Input: part model. Units: mm. Frame: model coordinates. A direction names the side the tool comes from. Coordinates: 2 decimals unless noted, no trailing zeros. Order: outer loops, then holes, each group sorted by start corner. A loop starts at its lowest first (then second) coordinate and runs counter-clockwise, first axis right, second up. Notation, with made-up numbers: M 62,43.5 L 91,43.5 A16 cw 91,64.5 Z; hole C 30,47.5 d9. An arc over 180 degrees is marked long. One line per item, written item: value.
```python
from build123d import *

# Parameters (mm, degrees)
F1_DEPTH    = 12
F2_T1_DEPTH = 22
F2_T3_DEPTH = 20.6602540378
F2_T5_DEPTH = 20.219219555
F2_T7_DEPTH = 19.7630643448
F3_SIZE     = 0.2


# Not quite as in the source:
# - a fillet or chamfer that OpenCascade refuses, or shapes differently, is made with other operations: its cross-section is extruded or revolved along the edge and cut away or added


with BuildPart() as f1:
    # F0 (on Top) → F1 (new body)
    with BuildSketch(Plane.XY):
        with BuildLine():
            Line((0, 17.1366985887), (0, 15.0604258217))
            Line((0, 15.0604258217), (-3, 15.0604258217))
            Line((-3, 15.0604258217), (-4, 17.0604258217))
            Line((-4, 17.0604258217), (-5, 17.0604258217))
            Line((-5, 17.0604258217), (-5, 10.4876235127))
            Line((-5, 10.4876235127), (-1.0879496576, 9.4864424318))
            ThreePointArc((-1.0879496576, 9.4864424318), (1.1165361393, 8.9993738808), (-1.0382550692, 8.3256764337))
            Line((-1.0382550692, 8.3256764337), (-5, 8.3256764337))
            Line((-5, 8.3256764337), (-5, 7.6356520876))
            Line((-5, 7.6356520876), (-5, 7.0604258217))
            Line((-5, 7.0604258217), (-3, 6.5184039995))
            Line((-3, 6.5184039995), (-3, 7.0604258217))
            Line((-3, 7.0604258217), (0, 7.0604258217))
            Line((0, 7.0604258217), (0, 5.0604258217))
            Line((0, 5.0604258217), (2.4494461788, 5.0604258217))
            Line((2.4494461788, 5.0604258217), (2.4494461788, 7.2136978708))
            ThreePointArc((2.4494461788, 7.2136978708), (4.7188246076, 13.8799594264), (11.0867818181, 16.8863264277))
            Line((11.0867818181, 16.8863264277), (15, 21.0604258217))
            Line((15, 21.0604258217), (2.1266145632, 21.0604258217))
            Line((2.1266145632, 21.0604258217), (0.7744232425, 21.0604258217))
            Line((0.7744232425, 21.0604258217), (0, 17.1366985887))
        make_face()
    extrude(amount=F1_DEPTH)

    # F2: fillet of radius 2 on 4 edges, made by hand

    # F2_s2 → F2_t1 (cut)
    with BuildSketch(Plane.XY.offset(-5)):
        with BuildLine():
            ThreePointArc((2.4494461788, 7.0604258217), (1.8636597412, 5.6462122593), (0.4494461788, 5.0604258217))
            Line((0.4494461788, 5.0604258217), (2.4494461788, 5.0604258217))
            Line((2.4494461788, 5.0604258217), (2.4494461788, 7.0604258217))
        make_face()
    extrude(amount=F2_T1_DEPTH, mode=Mode.SUBTRACT)

    # F2_s4 → F2_t3 (cut)
    with BuildSketch(Plane.XY.offset(-4.3301270189)):
        with BuildLine():
            ThreePointArc((-5, 15.3283750141), (-4.7320508076, 16.3283750141), (-4, 17.0604258217))
            Line((-4, 17.0604258217), (-5, 17.0604258217))
            Line((-5, 17.0604258217), (-5, 15.3283750141))
        make_face()
    extrude(amount=F2_T3_DEPTH, mode=Mode.SUBTRACT)

    # F2_s6 → F2_t5 (cut)
    with BuildSketch(Plane.XY.offset(-4.1096097775)):
        with BuildLine():
            ThreePointArc((2.4182671536, 21.0604258217), (1.1483331779, 20.6055043625), (0.4561194194, 19.4476935191))
            Line((0.4561194194, 19.4476935191), (0.7744232425, 21.0604258217))
            Line((0.7744232425, 21.0604258217), (2.4182671536, 21.0604258217))
        make_face()
    extrude(amount=F2_T5_DEPTH, mode=Mode.SUBTRACT)

    # F2_s8 → F2_t7 (cut)
    with BuildSketch(Plane.XY.offset(-3.8815321724)):
        with BuildLine():
            ThreePointArc((-3.4958636049, 10.1026814056), (-4.5798302456, 10.8138039967), (-5, 12.0402363817))
            Line((-5, 12.0402363817), (-5, 10.4876235127))
            Line((-5, 10.4876235127), (-3.4958636049, 10.1026814056))
        make_face()
    extrude(amount=F2_T7_DEPTH, mode=Mode.SUBTRACT)

    # F3
    f3_edges = [f1.edges().sort_by_distance(p)[0] for p in [
        (-3, 6.518404, 6),
    ]]
    chamfer(f3_edges, length=F3_SIZE)


solid = f1.part
```
(1) Cut plane C-C on y = 20. Output: boundary loops of the cut face in (x, z), plus the area to 3 significant figures.
Data:
outline: M 0.65,0 L 14.01,0 L 14.01,12 L 0.65,12 Z
area: 160 mm2
(2) Access query for faces 1 (the flat face through (-2, 7.06, 6)), 2 (the flat face through (0.23, 18.31, 5.92)), 3 (the cylindrical face through (-4.57, 10.8, 5.92)), 4 (the flat face through (-1, 15.06, 6)). Directions: +Z, -Z, +X, -X, +Y, -Y. A direction counts if a zero-diameter tool reaches every point of the face in a straight line with its end or side. Return the directions, or none.
Data:
face 1: +Z, -Z, -Y
face 2: +Z, -Z, -X, +Y
face 3: +Z, -Z, -X
face 4: +Z, -Z, +Y
(3) First-contact query: pin 1 (6 mm diameter, centred on y = 17, z = 9, fed in from -X); pin 2 (3 mm diameter, centred on x = 3, z = 3.5, fed in from -Y); pin 3 (3 mm diameter, centred on y = 18, z = 7, fed in from -X); pin 4 (2 mm diameter, centred on x = -0.05, y = 8.95, fed in from -Z). Flat tips, straight axial feed; report the tip coordinate or a pass-through.
Data:
pin 1: stops at x = -5
pin 2: stops at y = 5.36
pin 3: stops at x = -4.62
pin 4: passes through
(4) Ray query, line 1 (Y direction, x = 11, z = 5); line 2 (Y direction, x = -1, z = 5); line 3 (Y direction, x = -0.5, z = 1.75). Return the intervals inside material, ascending. Write a range as from..to.
Data:
line 1: y = 16.88..21.06
line 2: y = 7.06..8.27, 9.63..15.06
line 3: y = 7.06..7.87, 10.03..15.06
(5) Cut plane A-A on x = -1.5. Output: boundary loops of the cut face in (y, z), plus the area to 3 significant figures.
Data:
outline: M 7.06,0 L 8.33,0 L 8.33,12 L 7.06,12 Z; M 9.59,0 L 15.06,0 L 15.06,12 L 9.59,12 Z
area: 80.8 mm2
(6) Cut plane D-D on x = 12.25. Output: boundary loops of the cut face in (y, z).
Data:
outline: M 18.13,0 L 21.06,0 L 21.06,12 L 18.13,12 Z
(7) Draft query along X for faces 5 (the cylindrical face through (1.114, 9.042, 5.916)), 6 (the flat face through (3, 15, 0)), 7 (the cylindrical face through (1.163, 20.618, 5.916)). Return one class per face: released by +X, released by -X, zero draft, split by the parting line, or undercut.
Data:
face 5: undercut
face 6: zero draft
face 7: released by -X
(8) Cut plane B-B on z = 1.5. Output: boundary loops of the cut face in (x, y), plus the area to 3 significant figures.
Data:
outline: M -5,7.06 L -3.19,6.57 L -3,6.72 L -3,7.06 L 0,7.06 L 0,5.06 L 0.45,5.06 A2 ccw 2.45,7.06 L 2.45,7.21 A9.02 cw 11.09,16.89 L 15,21.06 L 2.42,21.06 A2 ccw 0.46,19.45 L 0,17.14 L 0,15.06 L -3,15.06 L -4,17.06 A2 ccw -5,15.33 L -5,12.04 A2 ccw -3.5,10.1 L -1.09,9.49 A1.17 cw long -1.04,8.33 L -5,8.33 Z
area: 130 mm2
